Geometry check sheet. Reference: the model listing, model coordinates, mm. A direction names the side the tool comes from. Give positions to 0.01 mm unless a question says otherwise; leave off trailing zeros. Write each loop counter-clockwise with the first axis right and the second up, starting at its lowest first coordinate (ties: lowest second). Pieces come first, ordered by that corner, then holes. Notation, with made-up numbers: M 78,-30 L 101,-30 A23 ccw 101,9 Z; hole C -22,-24.75 d6. An arc over 180 degrees is marked long. One line per item, written item: value. Start each with the question number.
1. Tool access check on faces 5 (the face through (-0.585, 1.972, -2.636)), 6 (the face through (1, 5, 1)). Record the directions out of +Z, -Z, +X, -X, +Y, -Y that give a thin tool (end or side, any length) a straight path to the whole face; none if there is none.
2. Release check for a two-part mould opening along Z. For faces 1 (the face through (-0.91, 4.51, 0.7)), 2 (the face through (-3.233, 2.465, 1.341)), 3 (the face through (-1, 0, -3)), 4 (the face through (1, 4, -1)) record: pulls with the +Z half, pulls with the -Z half, needs draft (parallel to the pull), parting line crosses it, or undercut.
3. Cross-section at A-A on x = 0. Record the cut outline in (y, z).
4. Cross-section at C-C on y = 3.1. Record the cut outline in (x, z).
5. Gauge pin test, flat ends, axial feed: pin 1 (2 mm diameter, centred on x = -2, y = 0.5, fed in from +Z); pin 2 (3 mm diameter, centred on y = 2, z = -1.5, fed in from -X); pin 3 (1.6 mm diameter, centred on x = 0, z = 0.5, fed in from -Y); pin 4 (3 mm diameter, centred on y = 2, z = -2.5, fed in from +X). Record the tip position at first contact, or that the pin passes through.
6. Cross-section at D-D on z = -2.5. Record the cut outline in (x, y).
7. Cross-section at B-B on z = 0. Record the cut outline in (x, y), then the cut area to 3 significant figures.
8. Scan lines: line 1 (Z direction, x = 0, y = 4.3); line 2 (Y direction, x = 2, z = 0.5); line 3 (Z direction, x = 0, y = 1.05). Record each from-to range of solid material in increasing order.
Autodesk Inventor part; units mm, degrees
ref_plane "YZ Plane" through (0, 0, 0) normal (1, 0, 0) x (0, 1, 0)
ref_plane "XZ Plane" through (0, 0, 0) normal (0, 1, 0) x (-1, 0, 0)
ref_plane "XY Plane" through (0, 0, 0) normal (0, 0, 1) x (1, 0, 0)
sketch "Sketch1" plane through (0, 0, 0) normal (0, 1, 0) x (-1, 0, 0)
  circle A0 centre (0, 0) radius 3.5
  dimension "d0" = 7
extrude "Extrusion1" add sketch "Sketch1" along normal blind 5
sketch "Sketch3" plane through (0, 0, 0) normal (0, -1, 0) x (1, 0, 0)
  circle A0 centre (0, 0) radius 2.7
  circle A1 centre (0, 0) radius 3.5
  dimension "d6" = 0.8
extrude "Extrusion3" cut sketch "Sketch3" against normal blind 4 contours A0
sketch "Sketch4" plane through (0, 5, 0) normal (0, 1, 0) x (1, 0, 0)
  circle A0 centre (0, 0) radius 2.7
  circle A1 centre (0, 0) radius 1.15
  dimension "d9" = 2.3
extrude "Extrusion4" cut sketch "Sketch4" against normal through all contours A1
properties part number "shaft endcap"
Report:
1. face 5: -Y
1. face 6: +Z, -Z, +X, -X, +Y
2. face 1: undercut
2. face 2: parting line crosses it
2. face 3: needs draft
2. face 4: undercut
3. outline: M 0,-3.5 L 5,-3.5 L 5,-1.15 L 4,-1.15 L 4,-2.7 L 0,-2.7 Z; M 0,2.7 L 4,2.7 L 4,1.15 L 5,1.15 L 5,3.5 L 0,3.5 Z
4. outline: C 0,0 d7; hole C 0,0 d5.4
5. pin 1: stops at z = 3.35
5. pin 2: stops at x = -3.5
5. pin 3: stops at y = 4
5. pin 4: stops at x = 3.35
6. outline: M -2.45,0 L -1.02,0 L -1.02,4 L 1.02,4 L 1.02,0 L 2.45,0 L 2.45,5 L -2.45,5 Z
7. outline: M -3.5,0 L -2.7,0 L -2.7,4 L -1.15,4 L -1.15,5 L -3.5,5 Z; M 1.15,4 L 2.7,4 L 2.7,0 L 3.5,0 L 3.5,5 L 1.15,5 Z
7. area: 11.1 mm^2
8. line 1: z = -3.5 to -1.15, 1.15 to 3.5
8. line 2: y = 4 to 5
8. line 3: z = -3.5 to -2.7, 2.7 to 3.5
